```python
from build123d import *

# Parameters (mm, degrees)
SKETCH1_R               = 3.175
BOSS_EXTRUDE1_DEPTH     = 152.4
CUT_EXTRUDE1_DEPTH      = 159.813487305
CUT_EXTRUDE1_DEPTH_BACK = 159.813487305
SKETCH3_R               = 1.4986


with BuildPart() as part:
    # Sketch1 → Boss-Extrude1 (new, symmetric)
    with BuildSketch(Plane(origin=(0, 0, 0), x_dir=(1, 0, 0), z_dir=(0, 1, 0))):
        with Locations(Location((0, 0, 0), (0, 0, 90))):
            Circle(SKETCH1_R)
    extrude(amount=BOSS_EXTRUDE1_DEPTH, both=True)

    # Sketch2 → Revolve1 (revolve)
    with BuildSketch(Plane.XY, mode=Mode.PRIVATE) as revolve1_sk:
        with BuildLine():
            Line((0, 158.75), (0, 152.4))
            Line((0, 152.4), (-3.175, 152.4))
            ThreePointArc((-3.175, 152.4), (-2.465048417, 152.838774209), (-2.54, 153.67))
            ThreePointArc((-2.54, 153.67), (-2.839806331, 156.994903166), (0, 158.75))
        make_face()
    revolve1 = revolve(revolve1_sk.sketch.rotate(Axis((0, 158.75, 0), (0, -1, 0)), 270), axis=Axis((0, 158.75, 0), (0, -1, 0)))

    # Mirror1: Revolve1 across plane
    add(revolve1.mirror(Plane.ZX))

    # Sketch3 → Cut-Extrude1 (cut, two sides: drawn at the far end of the back side and taken through both)
    with BuildSketch(Plane(origin=(0, 0, 0), x_dir=(1, 0, 0), z_dir=(0, 1, 0)).offset(-CUT_EXTRUDE1_DEPTH_BACK)):
        Circle(SKETCH3_R)
    extrude(amount=CUT_EXTRUDE1_DEPTH + CUT_EXTRUDE1_DEPTH_BACK, mode=Mode.SUBTRACT)


solid = part.part
```
Verification items for the finished model (mm, model axes). Coordinates: 2 decimals unless noted, no trailing zeros. Loops run counter-clockwise (first coordinate to the right, second up) from the corner with the lowest first, then second, coordinate; pieces in that order, holes last. Notation, with made-up numbers: (-13.5, 70.5) -> (-1.5, 70.5) arc R21 cw to (-1.5, 96.5) -> close; hole circle Ø4 at (41, 43.25). An arc over 180 degrees is marked (long way). Answer in a Markdown table with one row per item. Add a question column.
1. Material ranges on probe 1 along Y at (x, z) = (0.5, -2.5); probe 2 along Y at (x, z) = (-2.5, -1); probe 3 along X at (y, z) = (-20, 0) (3 decimals), recorded low to high. Write a range as [from, to].
2. Depth check by flat-ended pin: P1, Ø3, axis at y = -70.5, z = -2.5, coming from the -X side; P2, Ø2, axis at y = -45.5, z = -2, coming from the +X side. Enter the tip coordinate at first touch or a pass-through.
3. Section check C-C, the plane y = -70. Enter the section's corners in (x, z) (3 decimals).
Derived:
| question | item | result |
|---|---|---|
| 1 | probe 1 | y = [-157.47, -153.68], [-152.71, 152.71], [153.68, 157.47] |
| 1 | probe 2 | y = [-157.26, -153.89], [-152.56, 152.56], [153.89, 157.26] |
| 1 | probe 3 | x = [-3.175, -1.499], [1.499, 3.175] |
| 2 | P1 | stops at x = -3.01 |
| 2 | P2 | stops at x = 3.01 |
| 3 | outline | circle Ø6.35 at (0, 0); hole circle Ø2.997 at (0, 0) |
